Source: CAD feature listing. Evaluate the final solid. Frame: model axes, mm. A direction names the side the tool comes from. Round coordinates to 2 decimals unless told otherwise and drop trailing zeros. Loops run counter-clockwise (first coordinate to the right, second up) from the corner with the lowest first, then second, coordinate; pieces in that order, holes last.
(1) Section B-B, the plane x = -38. Return the cut outline in (y, z), plus the area to 3 significant figures.
(2) Mould query, pull axis Y, two halves, no side actions, for faces 1 (the flat face through (1, 1, 0)), 2 (the cylindrical face through (56.5, -28.9, 4.1)), 3 (the flat face through (-73.5, -28, 15)). Classes: pulls with the +Y half, pulls with the -Y half, needs draft (parallel to the pull), parting line crosses it, or undercut.
(3) Section C-C, the plane y = 18.5. Return the cut outline in (x, z), plus the area to 4 significant figures.
(4) Section D-D, the plane x = -68. Return the cut outline in (y, z), plus the area to 3 significant figures.
(5) Section A-A, the plane z = 23.5. Return the cut outline in (x, y).
(6) Material intervals for probe 1 along Y at (x, z) = (59.5, 6.7); probe 2 along X at (y, z) = (7, 2); probe 3 along Y at (x, z) = (54, 16.25), sorted ascending.
(7) Set-up query: faces 4 (the flat face through (-74.5, -1, 14)), 5 (the cylindrical face through (-72.49, -28.81, 11.58)), 6 (the flat face through (-64, -40, 15)). Return all of +Z, -Z, +X, -X, +Y, -Y with unobstructed straight access to the full face (end or side cutting, diameter ignored); none if empty.
(8) First-contact query: pin 1 Ø5 at (x, y) = (60, -30.5) entering from +Z; pin 2 Ø2 at (x, z) = (73.5, 12) entering from -Y; pin 3 Ø1.6 at (x, y) = (-59.5, 29) entering from +Z; pin 4 Ø2.5 at (x, y) = (-67.5, 43.5) entering from +Z. Flat tips, straight axial feed; report the tip coordinate or a pass-through.
```python
from build123d import *

# Parameters (mm, degrees)
PAD_DEPTH       = 29
SKETCH001_R     = 1.5
POCKET_DEPTH    = 28
SKETCH004_R     = 3
PAD001_DEPTH    = 6.3
SKETCH006_R     = 6.75
POCKET003_DEPTH = 5
SKETCH008_W     = 13.2
SKETCH008_H     = 8.5
POCKET005_DEPTH = 5
PAD002_DEPTH    = 3.5
SKETCH014_R     = 4.8
POCKET010_DEPTH = 1
SKETCH011_R     = 6.75
SKETCH011_R_2   = 5.25
POCKET011_DEPTH = 5
SKETCH015_R     = 4.4
POCKET012_DEPTH = 1
POCKET013_DEPTH = 5
SKETCH016_R     = 1
POCKET014_DEPTH = 3


with BuildPart() as part:
    # Sketch → Pad (new body)
    with BuildSketch(Plane.XY):
        with BuildLine():
            Line((-64.5, 49.5), (64.5, 49.5))
            ThreePointArc((74.5, 39.5), (71.571068, 46.571068), (64.5, 49.5))
            Line((74.5, 39.5), (74.5, -39.5))
            ThreePointArc((64.5, -49.5), (71.571068, -46.571068), (74.5, -39.5))
            Line((64.5, -49.5), (-64.5, -49.5))
            ThreePointArc((-74.5, -39.5), (-71.571068, -46.571068), (-64.5, -49.5))
            Line((-74.5, -39.5), (-74.5, 39.5))
            ThreePointArc((-64.5, 49.5), (-71.571068, 46.571068), (-74.5, 39.5))
        make_face()
    extrude(amount=PAD_DEPTH)

    # Sketch001 (on Face10 of Pad) → Pocket (cut)
    with BuildSketch(Plane.XY.offset(29)):
        with Locations((68, 43)):
            Circle(SKETCH001_R)
        with Locations((-68, 43)):
            Circle(SKETCH001_R)
        with Locations((68, -43)):
            Circle(SKETCH001_R)
        with Locations((-68, -43)):
            Circle(SKETCH001_R)
        Polygon((-57, 47), (57, 47), (72, 32), (72, -32), (57, -47), (-57, -47), (-72, -32), (-72, 32), align=None)
    extrude(amount=-POCKET_DEPTH, mode=Mode.SUBTRACT)

    # Sketch004 (on Face24 of Pocket) → Pad001 (join)
    with BuildSketch(Plane.XY.offset(1)):
        with Locations((-59.5, 29)):
            Circle(SKETCH004_R)
        with Locations((-59.5, -29)):
            Circle(SKETCH004_R)
        with Locations((59.5, -29)):
            Circle(SKETCH004_R)
        with Locations((59.5, 29)):
            Circle(SKETCH004_R)
    extrude(amount=PAD001_DEPTH)

    # Sketch006 (on Face7 of Pad001) → Pocket003 (cut)
    with BuildSketch(Plane(origin=(0, 49.5, 0), x_dir=(-1, 0, 0), z_dir=(0, 1, 0))):
        with Locations((-38, 13.5)):
            Circle(SKETCH006_R)
        with Locations((0, 13.5)):
            Circle(SKETCH006_R)
        with Locations((38, 13.5)):
            Circle(SKETCH006_R)
    extrude(amount=-POCKET003_DEPTH, mode=Mode.SUBTRACT)

    # Sketch008 (on Face9 of Pocket003) → Pocket005 (cut)
    with BuildSketch(Plane.YZ.offset(74.5)):
        with Locations((-23.6, 12.5)):
            Rectangle(SKETCH008_W, SKETCH008_H)
    extrude(amount=-POCKET005_DEPTH, mode=Mode.SUBTRACT)

    # Sketch010 → Pad002 (join)
    with BuildSketch(Plane.XY.offset(1)):
        Polygon((-47.65, 33.25), (-47.65, -33.25), (47.65, -33.25), (47.65, 33.25), (46.15, 33.25), (46.15, -31.75), (-46.15, -31.75), (-46.15, 33.25), align=None)
    extrude(amount=PAD002_DEPTH)

    # Sketch014 → Pocket010 (cut)
    with BuildSketch(Plane.YZ.offset(-72)):
        with Locations((-25, 14.5)):
            Circle(SKETCH014_R)
    extrude(amount=-POCKET010_DEPTH, mode=Mode.SUBTRACT)

    # Sketch011 → Pocket011 (cut)
    with BuildSketch(Plane.XZ.offset(49.5)):
        with Locations((0, 13.5)):
            Circle(SKETCH011_R)
        with Locations((38, 13.5)):
            Circle(SKETCH011_R)
        with Locations((-38, 13.5)):
            Circle(SKETCH011_R_2)
    extrude(amount=-POCKET011_DEPTH, mode=Mode.SUBTRACT)

    # Sketch015 → Pocket012 (cut)
    with BuildSketch(Plane(origin=(-74.5, 0, 0), x_dir=(0, -1, 0), z_dir=(-1, 0, 0))):
        with Locations((25, 14.5)):
            Circle(SKETCH015_R)
    extrude(amount=-POCKET012_DEPTH, mode=Mode.SUBTRACT)

    # Sketch012 → Pocket013 (cut)
    with BuildSketch(Plane(origin=(-74.5, 0, 0), x_dir=(0, -1, 0), z_dir=(-1, 0, 0))):
        with BuildLine():
            ThreePointArc((27.69875, 16.035808), (21.89485, 14.5), (27.69875, 12.964192))
            Line((27.69875, 16.035808), (27.69875, 12.964192))
        make_face()
    extrude(amount=-POCKET013_DEPTH, mode=Mode.SUBTRACT)

    # Sketch016 (on Face37 of Pocket013) → Pocket014 (cut)
    with BuildSketch(Plane.XY.offset(7.3)):
        with Locations((-59.5, 29)):
            Circle(SKETCH016_R)
        with Locations((-59.5, -29)):
            Circle(SKETCH016_R)
        with Locations((59.5, 29)):
            Circle(SKETCH016_R)
        with Locations((59.5, -29)):
            Circle(SKETCH016_R)
    extrude(amount=-POCKET014_DEPTH, mode=Mode.SUBTRACT)


solid = part.part
```
Output values:
1. outline: (-49.5, 0) - (49.5, 0) - (49.5, 6.75) - (47, 6.75) - (47, 1) - (-31.75, 1) - (-31.75, 4.5) - (-33.25, 4.5) - (-33.25, 1) - (-47, 1) - (-47, 8.25) - (-49.5, 8.25) - close; (-49.5, 18.75) - (-47, 18.75) - (-47, 29) - (-49.5, 29) - close; (47, 20.25) - (49.5, 20.25) - (49.5, 29) - (47, 29) - close
1. area: 184 mm2
2. face 1: needs draft
2. face 2: undercut
2. face 3: undercut
3. outline: (-74.5, 0) - (74.5, 0) - (74.5, 29) - (72, 29) - (72, 1) - (47.65, 1) - (47.65, 4.5) - (46.15, 4.5) - (46.15, 1) - (-46.15, 1) - (-46.15, 4.5) - (-47.65, 4.5) - (-47.65, 1) - (-72, 1) - (-72, 29) - (-74.5, 29) - close
3. area: 299.5 mm2
4. outline: (-48.87, 0) - (48.87, 0) - (48.87, 29) - (44.5, 29) - (44.5, 1) - (41.5, 1) - (41.5, 29) - (36, 29) - (36, 1) - (-36, 1) - (-36, 29) - (-41.5, 29) - (-41.5, 1) - (-44.5, 1) - (-44.5, 29) - (-48.87, 29) - close
4. area: 650 mm2
5. outline: (-74.5, -39.5) arc R10 ccw to (-64.5, -49.5) - (64.5, -49.5) arc R10 ccw to (74.5, -39.5) - (74.5, 39.5) arc R10 ccw to (64.5, 49.5) - (-64.5, 49.5) arc R10 ccw to (-74.5, 39.5) - close; hole (-72, -32) - (-57, -47) - (57, -47) - (72, -32) - (72, 32) - (57, 47) - (-57, 47) - (-72, 32) - close; hole circle Ø3 at (-68, -43); hole circle Ø3 at (-68, 43); hole circle Ø3 at (68, -43); hole circle Ø3 at (68, 43)
6. probe 1: y = -49.5 to -44.5, -32 to -30, -28 to -26, 26 to 28, 30 to 32, 44.5 to 49.5
6. probe 2: x = -74.5 to -72, -47.65 to -46.15, 46.15 to 47.65, 72 to 74.5
6. probe 3: y = -49.5 to -47, 47 to 49.5
7. face 4: +Z, -Z, -X, +Y, -Y
7. face 5: none
7. face 6: +Z
8. pin 1: stops at z = 7.3
8. pin 2: stops at y = -45.5
8. pin 3: stops at z = 4.3
8. pin 4: stops at z = 29
